Could you check a few things on this drawing? It's one solid part, dimensions in mm from its lowest x, y, z. A direction names the side the tool comes from. Coordinates: 2 decimals unless noted, no trailing zeros. Write each loop counter-clockwise with the first axis right and the second up, starting at its lowest first coordinate (ties: lowest second). Pieces come first, ordered by that corner, then holes. Notation, with made-up numbers: (84.5, -29) - (136.5, -29) arc R23 ccw to (136.5, -16) - close; hole circle Ø11 at (50, 33.5). An arc over 180 degrees is marked (long way). Use one line per item in the form item = value. Start each with the question number.
(1) If we section it at C-C on y = 1.25: Give the number of separate pieces and of enclosed holes in the cut face, then the cut area to 3 significant figures.
(2) If we section it at A-A on x = 7.5: Please give me the cut outline in (y, z).
(3) For pin 1 Ø1 at (x, y) = (56.5, 2) entering from -Z; pin 2 Ø1.9 at (y, z) = (2, 46.5) entering from +X; pin 3 Ø3 at (x, y) = (54, 4) entering from +Z; pin 4 Ø3 at (x, y) = (39.5, 3) entering from +Z, each with a flat end and sliding along its axis, tell me the tip position at first contact or that it passes through.
(4) If we section it at D-D on z = 37: Please give me the cut outline in (x, y).
(5) On a 3-axis mill with a long thin cutter (end or side, diameter ignored), from which of +Z, -Z, +X, -X, +Y, -Y can I reach the whole of each face in a straight line? I mean the marked faces 1, 2 and 3. Say none if no direction works.
(6) Thinking about a two-plate mould opening in Z: for the marked faces 4, 5 and 6, which applies, pulls with the +Z half, pulls with the -Z half, needs draft (parallel to the pull), parting line crosses it, or undercut?
(7) If I drill on probe 1 along X at (y, z) = (0.5, 60.5); probe 2 along Z at (x, y) = (56, 4.5); probe 3 along X at (y, z) = (4, 48), over which ranges is the centre line in solid material (lowest first)? Write a range as from..to.
(8) If we section it at B-B on z = 7: Please give me the cut outline in (x, y).
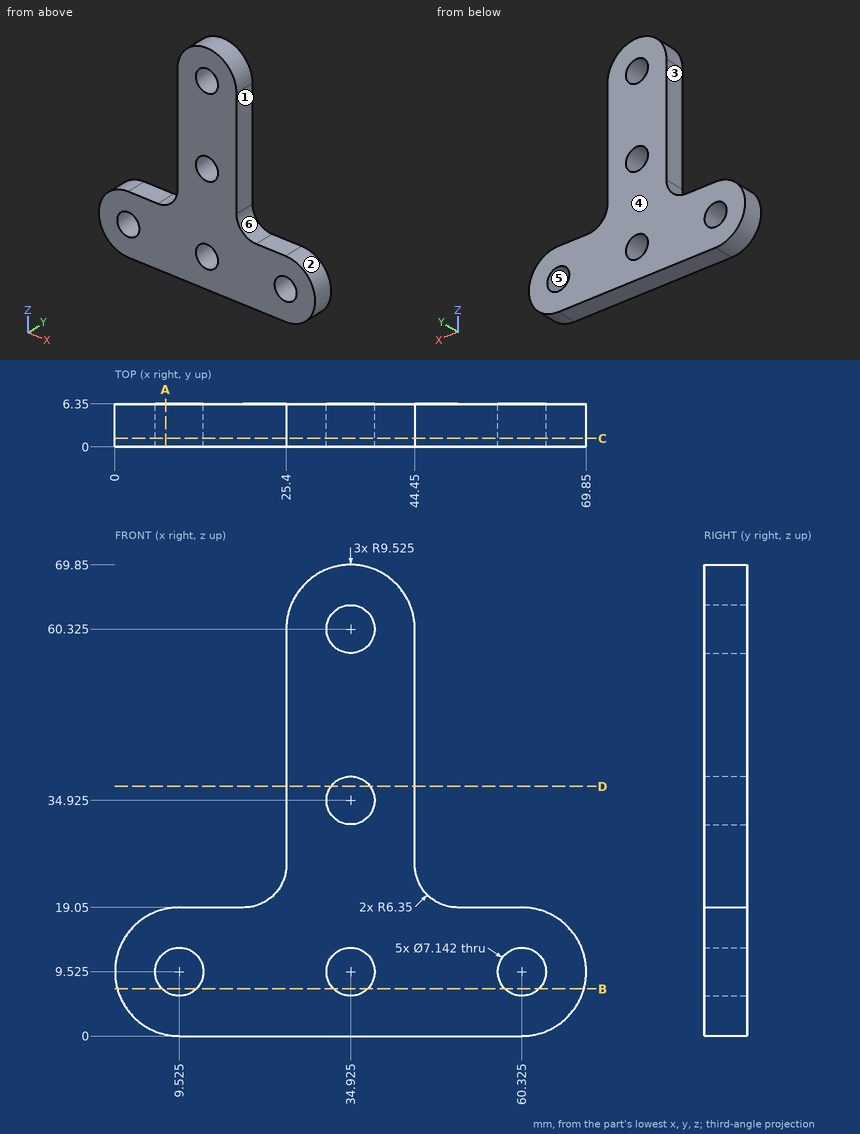
Reported:
q1.separate_pieces = 1
q1.enclosed_holes = 5
q1.area = 2,000 mm2
q2.outline = (0, 0.22) - (6.35, 0.22) - (6.35, 6.58) - (0, 6.58) - close; (0, 12.47) - (6.35, 12.47) - (6.35, 18.83) - (0, 18.83) - close
q3.pin_1 = 0
q3.pin_2 = 44.45
q3.pin_3 = 19.05
q3.pin_4 = 69.34
q4.outline = (25.4, 0) - (32.02, 0) - (32.02, 6.35) - (25.4, 6.35) - close; (37.83, 0) - (44.45, 0) - (44.45, 6.35) - (37.83, 6.35) - close
q5.face_1 = +Z, +X, +Y, -Y
q5.face_2 = +X, +Y, -Y
q5.face_3 = +Z, -X, +Y, -Y
q6.face_4 = needs draft
q6.face_5 = undercut
q6.face_6 = pulls with the +Z half
q7.probe_1 = 25.4..31.36, 38.49..44.45
q7.probe_2 = 0..19.05
q7.probe_3 = 25.4..44.45
q8.outline = (0.34, 0) - (7, 0) - (7, 6.35) - (0.34, 6.35) - close; (12.05, 0) - (32.4, 0) - (32.4, 6.35) - (12.05, 6.35) - close; (37.45, 0) - (57.8, 0) - (57.8, 6.35) - (37.45, 6.35) - close; (62.85, 0) - (69.51, 0) - (69.51, 6.35) - (62.85, 6.35) - close
